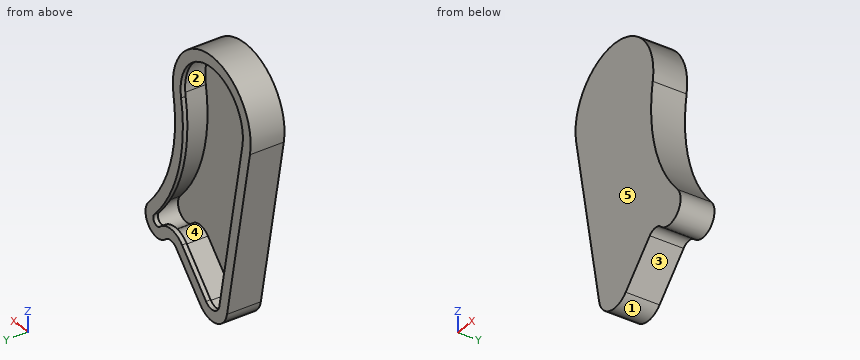
```python
from build123d import *

# Parameters (mm, degrees)
BOSS_EXTRUDE2_DEPTH = 15
CUT_EXTRUDE1_DEPTH  = 13
BOSS_EXTRUDE3_DEPTH = 2


with BuildPart() as part:
    # Sketch1 → Boss-Extrude2 (new body)
    with BuildSketch(Plane(origin=(0, 0, 0), x_dir=(1, 0, 0), z_dir=(0, 1, 0))):
        with BuildLine():
            Line((-24.556615071, 4.6875), (-9.822646028, 81.875))
            ThreePointArc((-9.822646028, 81.875), (-2.807110947, 89.597923116), (7.264280872, 86.872424857))
            Line((7.264280872, 86.872424857), (22.693183777, 70.563787572))
            ThreePointArc((22.693183777, 70.563787572), (26.210044162, 69.001329126), (29.795194528, 70.4))
            ThreePointArc((29.795194528, 70.4), (40.230934436, 70.374693007), (40.539091673, 59.943473184))
            ThreePointArc((40.539091673, 59.943473184), (26.07415519, 34.077117396), (24.595709122, 4.477844661))
            ThreePointArc((24.595709122, 4.477844661), (-0.106634546, -24.99977258), (-24.556615071, 4.6875))
        make_face()
    extrude(amount=BOSS_EXTRUDE2_DEPTH)

    # Sketch2 → Cut-Extrude1 (cut)
    with BuildSketch(Plane(origin=(0, 15, 0), x_dir=(1, 0, 0), z_dir=(0, 1, 0))):
        with BuildLine():
            Line((21.240327603, 69.1893026), (5.811424698, 85.497939885))
            ThreePointArc((5.811424698, 85.497939885), (-2.245688757, 87.678338492), (-7.858116823, 81.5))
            Line((-7.858116823, 81.5), (-22.592085865, 4.3125))
            ThreePointArc((-22.592085865, 4.3125), (-0.098103783, -22.999790774), (22.628052392, 4.119617088))
            ThreePointArc((22.628052392, 4.119617088), (24.151989109, 34.629636676), (39.06200056, 61.291880335))
            ThreePointArc((39.06200056, 61.291880335), (38.836018587, 68.941441539), (31.183142654, 68.96))
            ThreePointArc((31.183142654, 68.96), (26.163932142, 67.001860776), (21.240327603, 69.1893026))
        make_face()
    extrude(amount=-CUT_EXTRUDE1_DEPTH, mode=Mode.SUBTRACT)

    # Sketch3 → Boss-Extrude3 (add)
    with BuildSketch(Plane(origin=(0, 15, 0), x_dir=(1, 0, 0), z_dir=(0, 1, 0))):
        with BuildLine():
            Line((22.693183777, 70.563787572), (7.264280872, 86.872424857))
            ThreePointArc((7.264280872, 86.872424857), (-2.807110947, 89.597923116), (-9.822646028, 81.875))
            Line((-9.822646028, 81.875), (-24.556615071, 4.6875))
            ThreePointArc((-24.556615071, 4.6875), (-0.106634546, -24.99977258), (24.595709122, 4.477844661))
            ThreePointArc((24.595709122, 4.477844661), (26.07415519, 34.077117396), (40.539091673, 59.943473184))
            ThreePointArc((40.539091673, 59.943473184), (40.230934436, 70.374693007), (29.795194528, 70.4))
            ThreePointArc((29.795194528, 70.4), (26.210044162, 69.001329126), (22.693183777, 70.563787572))
        make_face()
        with BuildLine():
            Line((19.061043341, 67.127575143), (3.632140436, 83.436212428))
            ThreePointArc((3.632140436, 83.436212428), (-1.403555473, 84.798961558), (-4.911323014, 80.9375))
            Line((-4.911323014, 80.9375), (-19.645292057, 3.75))
            ThreePointArc((-19.645292057, 3.75), (-0.085307637, -19.999818064), (19.676567297, 3.582275729))
            ThreePointArc((19.676567297, 3.582275729), (21.268739987, 35.458415597), (36.846363891, 63.314491061))
            ThreePointArc((36.846363891, 63.314491061), (36.743644812, 66.791564336), (33.265064843, 66.8))
            ThreePointArc((33.265064843, 66.8), (26.094764111, 64.002658251), (19.061043341, 67.127575143))
        make_face(mode=Mode.SUBTRACT)
    extrude(amount=-BOSS_EXTRUDE3_DEPTH)


solid = part.part
```
The listing builds one solid part. Answer for the finished solid, in the listing's coordinates (mm). Face numbers are marked on the shaded views. A direction names the side the tool comes from. Coordinates: 2 decimals unless noted, no trailing zeros. Loops run counter-clockwise (first coordinate to the right, second up) from the corner with the lowest first, then second, coordinate; pieces in that order, holes last. Notation, with made-up numbers: (1.5, 61.5) - (48.5, 61.5) arc R6 cw to (48.5, 68.5) - close; hole circle Ø2 at (10.25, 26.25). An arc over 180 degrees is marked (long way). Use a Markdown table: item, result. Add a question column.
1) Find the intervals of material crossed by line 1 (X direction, y = 14.3, z = 0); line 2 (Y direction, x = 29, z = -49); line 3 (Z direction, x = 0, y = 13.4), in increasing order.
2) The mould has two halves that part along Y. Classify the marked faces 3, 4 and 5: released by +Y, released by -Y, zero draft, split by the parting line, or undercut.
3) Given pin 1 (4 mm diameter, centred on x = 17, z = -26.5, fed in from +Y); pin 2 (1 mm diameter, centred on y = 11.5, z = 11.5, fed in from +X); pin 3 (3 mm diameter, centred on x = 7, y = 6.5, fed in from +Z), each flat-ended and moving along its own axis, determine where each tip first touches the part or whether it passes through.
4) The part is cut by section B-B, the plane y = 7.25. Give the vertices of the cut face in (x, z) (1 decimal), and give its area (3 significant figures).
5) The part is cut by section A-A, the plane z = 0. Give the vertices of the cut face in (x, y), and give its area (3 significant figures).
6) For the marked faces 1 and 2, determine the directions among +Z, -Z, +X, -X, +Y, -Y from which every point of the face is accessible in a straight line to the end or side of a thin tool.
7) The part is cut by section C-C, the plane x = 0. Give the vertices of the cut face in (y, z).
Here are the results:
| question | item | result |
|---|---|---|
| 1 | line 1 | x = -25 to -20, 20 to 25 |
| 1 | line 2 | y = 0 to 2, 13 to 15 |
| 1 | line 3 | z = -90 to -85, 20 to 25 |
| 2 | face 3 | zero draft |
| 2 | face 4 | undercut |
| 2 | face 5 | released by -Y |
| 3 | pin 1 | stops at y = 2 |
| 3 | pin 2 | stops at x = 22.45 |
| 3 | pin 3 | stops at z = 24.39 |
| 4 | outline | (-24.6, -4.7) - (-9.8, -81.9) arc R10 ccw to (7.3, -86.9) - (22.7, -70.6) arc R5 cw to (29.8, -70.4) arc R7.5 ccw to (40.5, -59.9) arc R65 cw to (24.6, -4.5) arc R25 ccw (long way) to start; hole (-22.6, -4.3) - (-7.9, -81.5) arc R8 ccw to (5.8, -85.5) - (21.2, -69.2) arc R7 cw to (31.2, -69) arc R5.5 ccw to (39.1, -61.3) arc R67 cw to (22.6, -4.1) arc R23 ccw (long way) to start |
| 4 | area | 590 mm^2 |
| 5 | outline | (-25, 0) - (25, 0) - (25, 15) - (20, 15) - (20, 13) - (23, 13) - (23, 2) - (-23, 2) - (-23, 13) - (-20, 13) - (-20, 15) - (-25, 15) - close |
| 5 | area | 164 mm^2 |
| 6 | face 1 | -Z, +Y, -Y |
| 6 | face 2 | none |
| 7 | outline | (0, -90) - (15, -90) - (15, -85) - (13, -85) - (13, -88) - (2, -88) - (2, 23) - (13, 23) - (13, 20) - (15, 20) - (15, 25) - (0, 25) - close |
